```python
from build123d import *

# Parameters (mm, degrees)
F4_DEPTH     = 1.5875
F0_W         = 1.4224
F0_H         = 12.7
F5_DEPTH     = 25.4
F1_R         = 0.87629
F2_DEPTH     = 25.4
F7_T1_DEPTH  = 1.7526
F7_T6_DEPTH  = 12.9686376242
F7_T12_DEPTH = 12.9686376242
F7_T17_DEPTH = 10.3818412391


# Not quite as in the source:
# - a fillet or chamfer that OpenCascade refuses, or shapes differently, is made with other operations: its cross-section is extruded or revolved along the edge and cut away or added
# - a fillet or chamfer is up to 0.001 mm smaller than in the source, because OpenCascade refuses the exact size


with BuildPart() as f4:
    # F3 (on Right) → F4 (new body, symmetric)
    with BuildSketch(Plane.YZ):
        Polygon((35.5477839421, -4.7625), (38.1, 4.7625), (-38.1, 4.7625), (-38.1, -4.7625), align=None)
    extrude(amount=F4_DEPTH, both=True)

    # F0 (on face) → F5 (cut)
    with BuildSketch(Plane.XY.offset(4.7625)):
        with Locations((-0.8763, 31.75)):
            Rectangle(F0_W, F0_H)
    extrude(amount=-F5_DEPTH, mode=Mode.SUBTRACT)

    # F1 (radius 0.8763 in the source; OpenCascade refuses exactly that, so slightly less here)
    f1_edges = [f4.edges().sort_by_distance(p)[0] for p in [
        (1.5875, 36.823892, 0),
        (-0.1651, 36.823892, 0),
    ]]
    fillet(f1_edges, radius=F1_R)

    # F6 (on face) → F2 (cut)
    with BuildSketch(Plane.YZ.offset(1.5875)):
        Polygon((37.1927978359, 4.7625), (25.4, 4.7625), (25.4, 1.5875), (36.6047261297, 2.5677865143), align=None)
        Polygon((43.6932000767, 4.7625), (37.1927978359, 4.7625), (36.6047261297, 2.5677865143), (43.6932000767, 3.1879476263), align=None)
    extrude(amount=-F2_DEPTH, mode=Mode.SUBTRACT)

    # F7: fillet of radius 3.175 on 2 edges, made by hand

    # F7_s2 → F7_t1 (join)
    with BuildSketch(Plane.YZ.offset(-0.1651)):
        with BuildLine():
            ThreePointArc((25.4, 4.7625), (26.5256229175, 2.6151836003), (28.8385617484, 1.8883351718))
            Line((28.8385617484, 1.8883351718), (25.4, 1.5875))
            Line((25.4, 1.5875), (25.4, 4.7625))
        make_face()
    extrude(amount=F7_T1_DEPTH)


with BuildPart() as f7_tool4:
    # F7_s5 → F7_t6 (new body)
    with BuildSketch(Plane.XY.offset(8.2061376242)):
        with BuildLine():
            ThreePointArc((-0.1651, 28.0474550497), (-0.5432151257, 26.5447707848), (-1.5875, 25.4))
            Line((-1.5875, 25.4), (-0.1651, 25.4))
            Line((-0.1651, 25.4), (-0.1651, 28.0474550497))
        make_face()
    extrude(amount=-F7_T6_DEPTH)

    split(bisect_by=Plane(origin=(0, 0.0551082957, -0.6298907024), x_dir=(1, 0, 0), z_dir=(0, 0.0871557427, -0.9961946981)), keep=Keep.TOP)


with BuildPart() as f4_1:
    add(f4.part)

    # F7_t3: union F7_tool4
    add(f7_tool4.part)


with BuildPart() as f7_tool10:
    # F7_s11 → F7_t12 (new body)
    with BuildSketch(Plane.XY.offset(8.2061376242)):
        with BuildLine():
            ThreePointArc((-0.1651, 28.0474550497), (-0.5432151257, 26.5447707848), (-1.5875, 25.4))
            Line((-1.5875, 25.4), (-0.1651, 25.4))
            Line((-0.1651, 25.4), (-0.1651, 28.0474550497))
        make_face()
    extrude(amount=-F7_T12_DEPTH)

    split(bisect_by=Plane.XY.offset(4.7625), keep=Keep.BOTTOM)

    split(bisect_by=Plane(origin=(0, 0.0551082957, -0.6298907024), x_dir=(1, 0, 0), z_dir=(0, -0.0871557427, 0.9961946981)), keep=Keep.TOP)


with BuildPart() as f7_tool15:
    # F7_s16 → F7_t17 (new body)
    with BuildSketch(Plane.YZ.offset(1.5875)):
        with BuildLine():
            ThreePointArc((25.4, 4.7625), (26.5256229175, 2.6151836003), (28.8385617484, 1.8883351718))
            Line((28.8385617484, 1.8883351718), (25.4, 1.5875))
            Line((25.4, 1.5875), (25.4, 4.7625))
        make_face()
    extrude(amount=-F7_T17_DEPTH)

    split(bisect_by=Plane.YZ.offset(-0.1651), keep=Keep.BOTTOM)

    split(bisect_by=Plane.YZ.offset(-1.5875), keep=Keep.TOP)


with BuildPart() as f7_tool10_1:
    add(f7_tool10.part)

    # F7_t20: intersect F7_tool15
    add(f7_tool15.part, mode=Mode.INTERSECT)


with BuildPart() as f4_2:
    add(f4_1.part)

    # F7_t8: union F7_tool10
    add(f7_tool10_1.part)


solid = f4_2.part
```
Here's how the part is built. I have some questions about the finished solid (model axes, mm). A direction names the side the tool comes from. Round coordinates to 2 decimals unless told otherwise and drop trailing zeros. Order: outer loops, then holes, each group sorted by start corner. A loop starts at its lowest first (then second) coordinate and runs counter-clockwise, first axis right, second up. Notation, with made-up numbers: M -30.75,24.25 L -26.75,24.25 A13 cw -26.75,38.25 Z; hole C -9,45.25 d4. An arc over 180 degrees is marked long. One line per question, with ' | ' between items.
1) I need wall thicknesses on line 1 along Y through (x, z) = (-0.8, -3.75); line 2 along Y through (x, z) = (0.1, 3.25); line 3 along Z through (x, y) = (0.35, 34). Which ranges of each line are inside material? Lowest first, please.
Working result:
line 1: -38.1 to 26.14 | line 2: -38.1 to 25.95 | line 3: -4.76 to 2.34
2) If we mould it in two halves opening along Y, with no side actions, what happens to faces 1 (the face through (0, -1, -4.762)), 2 (the face through (0.375, 26.112, 3.032)), 3 (the face through (-0.533, 26.564, -0.992))? For each: +Y half, -Y half, draft (parallel to the pull), parting line (faces both ways), or undercut.
Working result:
face 1: draft | face 2: undercut | face 3: +Y half
3) For pin 1 Ø2 at (y, z) = (31, -1.5) entering from -X, with a flat end and sliding along its axis, tell me the tip position at first contact or that it passes through.
Working result:
pin 1: x = -0.17
4) For faces 4 (the face through (1.588, 0, 0)), 5 (the face through (-0.165, 32, -1)), which set-ups out of +Z, -Z, +X, -X, +Y, -Y let a thin tool reach every point of the face, with its end or its side?
Working result:
face 4: +Z, -Z, +X, +Y, -Y | face 5: +Z, -Z, -X, +Y
5) I want a section at B-B, the plane y = 31. Write out the boundary of the cut face in (x, z), then the cut area to 3 significant figures.
Working result:
outline: M -0.17,-4.76 L 1.59,-4.76 L 1.59,2.08 L -0.17,2.08 Z | area: 12.0 mm²
